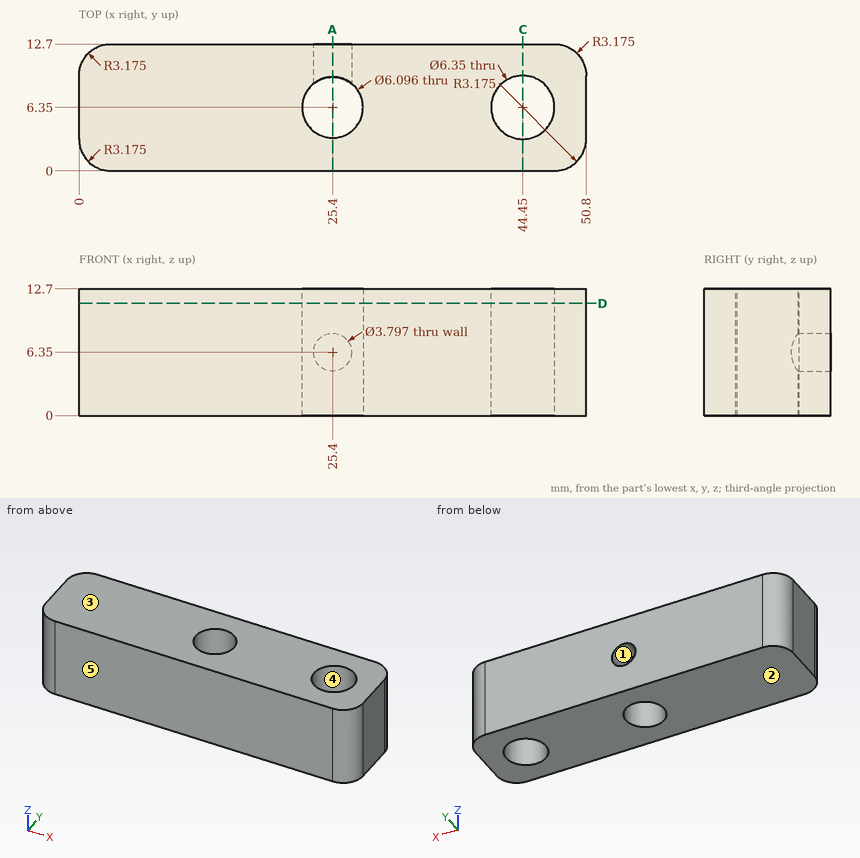
Answer from the drawing. Dimensions are ordinates in mm from the lowest x, y and z of the part. A direction names the side the tool comes from. Round coordinates to 2 decimals unless told otherwise and drop trailing zeros. Loops run counter-clockwise (first coordinate to the right, second up) from the corner with the lowest first, then second, coordinate; pieces in that order, holes last. Notation, with made-up numbers: (75, 34) - (84, 34) arc R9 cw to (84, 44) - close; hole circle Ø6 at (31.25, 49). An arc over 180 degrees is marked (long way). One line per item, written item: value.
Q1. Find section D-D on z = 11.25. State how many separate pieces and enclosed holes the cut face has, and give its area (3 significant figures).
Check values:
separate pieces: 1
enclosed holes: 2
area: 576 mm2
Q2. Find section C-C on x = 44.45. Give the vertices of the cut face in (y, z) (1 decimal).
Check values:
outline: (0, 0) - (3.2, 0) - (3.2, 12.7) - (0, 12.7) - close; (9.5, 0) - (12.7, 0) - (12.7, 12.7) - (9.5, 12.7) - close
Q3. Find section A-A on x = 25.4. Give the vertices of the cut face in (y, z).
Check values:
outline: (0, 0) - (3.3, 0) - (3.3, 12.7) - (0, 12.7) - close; (9.4, 0) - (12.7, 0) - (12.7, 4.45) - (9.4, 4.45) - close; (9.4, 8.25) - (12.7, 8.25) - (12.7, 12.7) - (9.4, 12.7) - close
Q4. Each of these flat-tipped pins is pushed along its axis until it touches: pin 1 Ø5 at (x, y) = (24, 7.5) entering from -Z; pin 2 Ø3.5 at (x, y) = (25.4, 6.35) entering from +Z. Where does it stop, or does it pass through?
Check values:
pin 1: z = 0
pin 2: through
Q5. For the marked faces 1 and 2, determine the directions among +Z, -Z, +X, -X, +Y, -Y from which every point of the face is accessible in a straight line to the end or side of a thin tool.
Check values:
face 1: +Y
face 2: -Z, +X, -X, +Y, -Y
Q6. Straight lines are drawn through the part: probe 1 along X at (y, z) = (6.5, 7.25); probe 2 along Y at (x, z) = (44.45, 3.75) (1 decimal); probe 3 along Z at (x, y) = (25.4, 11.05). For each, find the intervals that lie inside material, in ascending order.
Check values:
probe 1: 0 to 22.36, 28.44 to 41.28, 47.62 to 50.8
probe 2: 0 to 3.2, 9.5 to 12.7
probe 3: 0 to 4.45, 8.25 to 12.7
Q7. The mould has two halves that part along Y. Classify the marked faces 3, 4 and 5: +Y half, -Y half, draft (parallel to the pull), parting line (faces both ways), or undercut.
Check values:
face 3: draft
face 4: undercut
face 5: -Y half
